Verification items for the finished model (mm, model axes). A direction names the side the tool comes from. Coordinates: 2 decimals unless noted, no trailing zeros. Write each loop counter-clockwise with the first axis right and the second up, starting at its lowest first coordinate (ties: lowest second). Pieces come first, ordered by that corner, then holes. Notation, with made-up numbers: (70.5, 53) -> (95.5, 53) arc R15 ccw to (95.5, 68) -> close; hole circle Ø4 at (-8.5, 76). An arc over 180 degrees is marked (long way). Answer in a Markdown table with one row per item.
```python
from build123d import *

# Parameters (mm, degrees)
SKETCH1_W           = 32
SKETCH1_H           = 32
SKETCH1_R           = 3.02
SKETCH1_R_2         = 1.7
BOSS_EXTRUDE1_DEPTH = 9.864848297
SKETCH1_5_R         = 9
CUT_EXTRUDE2_DEPTH  = 2
SKETCH7_W           = 32
SKETCH7_H           = 9.864848297
BOSS_EXTRUDE3_DEPTH = 17.613942208
SKETCH10_W          = 17.613942208
SKETCH10_H          = 32
BOSS_EXTRUDE5_DEPTH = 32
SKETCH11_R          = 1.7
CUT_EXTRUDE3_DEPTH  = 49


with BuildPart() as part:
    # Sketch1 → Boss-Extrude1 (new body)
    with BuildSketch(Plane(origin=(0, 0, 0), x_dir=(1, 0, 0), z_dir=(0, 1, 0))):
        Rectangle(SKETCH1_W, SKETCH1_H)
        with Locations(Location((0, 0, 0), (0, 0, 270))):
            Circle(SKETCH1_R, mode=Mode.SUBTRACT)
        with Locations(Location((0, 11, 0), (0, 0, 270))):
            Circle(SKETCH1_R_2, mode=Mode.SUBTRACT)
        with Locations(Location((-11, 0, 0), (0, 0, 270))):
            Circle(SKETCH1_R_2, mode=Mode.SUBTRACT)
        with Locations(Location((0, -11, 0), (0, 0, 270))):
            Circle(SKETCH1_R_2, mode=Mode.SUBTRACT)
        with Locations(Location((11, 0, 0), (0, 0, 270))):
            Circle(SKETCH1_R_2, mode=Mode.SUBTRACT)
    extrude(amount=-BOSS_EXTRUDE1_DEPTH)

    # Sketch1_5 → Cut-Extrude2 (cut)
    with BuildSketch(Plane(origin=(0, 0, 0), x_dir=(1, 0, 0), z_dir=(0, 1, 0))):
        with Locations(Location((0, 0, 0), (0, 0, 270))):
            Circle(SKETCH1_5_R)
    extrude(amount=-CUT_EXTRUDE2_DEPTH, mode=Mode.SUBTRACT)

    # Sketch7 → Boss-Extrude3 (add)
    with BuildSketch(Plane(origin=(16, 0, 0), x_dir=(0, 0, -1), z_dir=(1, 0, 0))):
        with Locations((0, -4.932424148)):
            Rectangle(SKETCH7_W, SKETCH7_H)
    extrude(amount=BOSS_EXTRUDE3_DEPTH)

    # Sketch10 → Boss-Extrude5 (add)
    with BuildSketch(Plane(origin=(0, 0, 0), x_dir=(1, 0, 0), z_dir=(0, 1, 0))):
        with Locations((24.806971104, 0)):
            Rectangle(SKETCH10_W, SKETCH10_H)
    extrude(amount=BOSS_EXTRUDE5_DEPTH)

    # Sketch11 → Cut-Extrude3 (cut, through all)
    with BuildSketch(Plane.ZY.offset(-16)):
        with Locations((-7.778174593, 23.778174593)):
            Circle(SKETCH11_R)
        with Locations((7.778174593, 23.778174593)):
            Circle(SKETCH11_R)
        with Locations((7.778174593, 8.221825407)):
            Circle(SKETCH11_R)
        with Locations((-7.778174593, 8.221825407)):
            Circle(SKETCH11_R)
    extrude(amount=-CUT_EXTRUDE3_DEPTH, mode=Mode.SUBTRACT)


solid = part.part
```
1. Mould release check, pull along Y, two halves, no side actions. Record for faces 4 (the cylindrical face through (24.68, 22.27, 8.56)), 5 (the flat face through (-7, 0, 7)), 6 (the flat face through (33.614, 11, 0)): released by +Y, released by -Y, zero draft, split by the parting line, or undercut.
Geometry says:
| item | result |
|---|---|
| face 4 | undercut |
| face 5 | released by +Y |
| face 6 | zero draft |
2. Section check D-D, the plane z = -11. Record the boundary of the cut face in (x, y), plus the area to 3 significant figures.
Geometry says:
| item | result |
|---|---|
| outline | (-16, -9.86) -> (-1.7, -9.86) -> (-1.7, 0) -> (-16, 0) -> close; (1.7, -9.86) -> (33.61, -9.86) -> (33.61, 32) -> (16, 32) -> (16, 0) -> (1.7, 0) -> close |
| area | 1,020 mm^2 |
3. Tool access check on faces 1 (the flat face through (16, 16, 0)), 2 (the cylindrical face through (0.51, -4.86, 12.62)), 3 (the cylindrical face through (2.703, -0.986, 8.584)). Record the directions out of +Z, -Z, +X, -X, +Y, -Y that give a thin tool (end or side, any length) a straight path to the whole face; none if there is none.
Geometry says:
| item | result |
|---|---|
| face 1 | +Z, -Z, -X, +Y |
| face 2 | +Y, -Y |
| face 3 | +Y |
4. Section check B-B, the plane x = 0. Record the boundary of the cut face in (y, z).
Geometry says:
| item | result |
|---|---|
| outline | (-9.86, -16) -> (0, -16) -> (0, -12.7) -> (-9.86, -12.7) -> close; (-9.86, -9.3) -> (0, -9.3) -> (0, -9) -> (-2, -9) -> (-2, -3.02) -> (-9.86, -3.02) -> close; (-9.86, 3.02) -> (-2, 3.02) -> (-2, 9) -> (0, 9) -> (0, 9.3) -> (-9.86, 9.3) -> close; (-9.86, 12.7) -> (0, 12.7) -> (0, 16) -> (-9.86, 16) -> close |
5. Section check A-A, the plane z = 0. Record the boundary of the cut face in (x, y).
Geometry says:
| item | result |
|---|---|
| outline | (-16, -9.86) -> (-12.7, -9.86) -> (-12.7, 0) -> (-16, 0) -> close; (-9.3, -9.86) -> (-3.02, -9.86) -> (-3.02, -2) -> (-9, -2) -> (-9, 0) -> (-9.3, 0) -> close; (3.02, -9.86) -> (9.3, -9.86) -> (9.3, 0) -> (9, 0) -> (9, -2) -> (3.02, -2) -> close; (12.7, -9.86) -> (33.61, -9.86) -> (33.61, 32) -> (16, 32) -> (16, 0) -> (12.7, 0) -> close |
6. Depth check by flat-ended pin: P1, Ø2.5, axis at x = -11, z = 0, coming from the +Y side; P2, Ø10, axis at x = -9, z = -4, coming from the +Y side; P3, Ø6, axis at y = 6.5, z = -4.5, coming from the -X side; P4, Ø5.5, axis at x = 0, z = -11, coming from the -Y side. Enter the tip coordinate at first touch or a pass-through.
Geometry says:
| item | result |
|---|---|
| P1 | through |
| P2 | y = 0 |
| P3 | x = 16 |
| P4 | y = -9.86 |
7. Section check C-C, the plane x = 11. Record the boundary of the cut face in (y, z), plus the area to 3 significant figures.
Geometry says:
| item | result |
|---|---|
| outline | (-9.86, -16) -> (0, -16) -> (0, -1.7) -> (-9.86, -1.7) -> close; (-9.86, 1.7) -> (0, 1.7) -> (0, 16) -> (-9.86, 16) -> close |
| area | 282 mm^2 |
8. Thickness scan on line 1 (X direction, y = -6.5, z = 0); line 2 (X direction, y = -4, z = 1); line 3 (Z direction, x = -0.5, y = -5). Record the ranges inside material, lowest first. Write a range as from..to.
Geometry says:
| item | result |
|---|---|
| line 1 | -16..-12.7, -9.3..-3.02, 3.02..9.3, 12.7..33.61 |
| line 2 | -16..-12.37, -9.63..-2.85, 2.85..9.63, 12.37..33.61 |
| line 3 | -16..-12.62, -9.38..-2.98, 2.98..9.38, 12.62..16 |
